```python
from build123d import *

# Parameters (mm, degrees)
BOSS_EXTRUDE1_DEPTH = 3


with BuildPart() as part:
    # Sketch1 → Boss-Extrude1 (new body)
    with BuildSketch(Plane.XY):
        Polygon((-70, -236), (70, -236), (70, -233), (56.25, -88), (56.25, 45), (-56.25, 45), (-56.25, -88), (-70, -233), align=None)
        with BuildLine():
            Line((40, -16), (-40, -16))
            ThreePointArc((-40, -16), (-45, -21), (-40, -26))
            Line((-40, -26), (40, -26))
            ThreePointArc((40, -26), (45, -21), (40, -16))
        make_face(mode=Mode.SUBTRACT)
        with BuildLine():
            Line((25, 15), (25, 25))
            Line((25, 25), (-25, 25))
            Line((-25, 25), (-25, 15))
            Line((-25, 15), (-4, 15))
            Line((-4, 15), (-4, 0))
            ThreePointArc((-4, 0), (0, -4), (4, 0))
            Line((4, 0), (4, 15))
            Line((4, 15), (25, 15))
        make_face(mode=Mode.SUBTRACT)
        with BuildLine():
            Line((40, -41), (-40, -41))
            ThreePointArc((-40, -41), (-52, -53), (-40, -65))
            Line((-40, -65), (40, -65))
            ThreePointArc((40, -65), (52, -53), (40, -41))
        make_face(mode=Mode.SUBTRACT)
        with BuildLine():
            Line((40, -80), (-40, -80))
            ThreePointArc((-40, -80), (-52, -92), (-40, -104))
            Line((-40, -104), (40, -104))
            ThreePointArc((40, -104), (52, -92), (40, -80))
        make_face(mode=Mode.SUBTRACT)
        with BuildLine():
            Line((40, -119), (-40, -119))
            ThreePointArc((-40, -119), (-52, -131), (-40, -143))
            Line((-40, -143), (40, -143))
            ThreePointArc((40, -143), (52, -131), (40, -119))
        make_face(mode=Mode.SUBTRACT)
        with BuildLine():
            Line((42.5, -158), (-42.5, -158))
            ThreePointArc((-42.5, -158), (-54.5, -170), (-42.5, -182))
            Line((-42.5, -182), (42.5, -182))
            ThreePointArc((42.5, -182), (54.5, -170), (42.5, -158))
        make_face(mode=Mode.SUBTRACT)
        with BuildLine():
            Line((45, -197), (-45, -197))
            ThreePointArc((-45, -197), (-57, -209), (-45, -221))
            Line((-45, -221), (45, -221))
            ThreePointArc((45, -221), (57, -209), (45, -197))
        make_face(mode=Mode.SUBTRACT)
    extrude(amount=BOSS_EXTRUDE1_DEPTH)


solid = part.part
```
Geometry check sheet. Reference: the model listing, model coordinates, mm. A direction names the side the tool comes from. Coordinates: 2 decimals unless noted, no trailing zeros. Loops run counter-clockwise (first coordinate to the right, second up) from the corner with the lowest first, then second, coordinate; pieces in that order, holes last. Notation, with made-up numbers: (29, 32) - (74, 32) arc R16 ccw to (74, 55) - close; hole circle Ø8 at (14.25, -0.75). An arc over 180 degrees is marked (long way). One line per item, written item: value. Start each with the question number.
(1) Depth check by flat-ended pin: P1, Ø0.9, axis at y = 22.5, z = 2, coming from the -X side. Enter the tip coordinate at first touch or a pass-through.
(2) Mould release check, pull along X, two halves, no side actions. Record for faces 1 (the cylindrical face through (52, -131, 1)), 2 (the flat face through (-1, -31, 3)), 3 (the flat face through (63.22, -161.51, 1.48)): released by +X, released by -X, zero draft, split by the parting line, or undercut.
(3) Tool access check on faces 4 (the flat face through (-63.03, -159.49, 1.48)), 5 (the cylindrical face through (-52, -92, 1)). Record the directions out of +Z, -Z, +X, -X, +Y, -Y that give a thin tool (end or side, any length) a straight path to the whole face; none if there is none.
(4) Cross-section at B-B on z = 2.3. Count the separate pieces of the cut face and the enclosed holes in it, plus the area to 3 significant figures.
(5) Cross-section at D-D on y = -33. Enter the section's corners in (x, z).
(6) Cross-section at C-C on y = -131. Enter the section's corners in (x, z).
(7) Material ranges on line 1 (Y direction, x = 47, z = 2.7); line 2 (Y direction, x = 51, z = 2.2); line 3 (X direction, y = -159, z = 2.3), recorded low to high. Write a range as [from, to].
(8) Cross-section at A-A on y = 8.5. Enter the section's corners in (x, z), plus the area to 4 significant figures.
Results below:
1. P1: stops at x = -56.25
2. face 1: undercut
2. face 2: zero draft
2. face 3: released by +X
3. face 4: +Z, -Z, -X, +Y
3. face 5: +Z, -Z
4. separate pieces: 1
4. enclosed holes: 7
4. area: 19,900 mm2
5. outline: (-56.25, 0) - (56.25, 0) - (56.25, 3) - (-56.25, 3) - close
6. outline: (-60.33, 0) - (-52, 0) - (-52, 3) - (-60.33, 3) - close; (52, 0) - (60.33, 0) - (60.33, 3) - (52, 3) - close
7. line 1: y = [-236, -220.83], [-197.17, -181.12], [-158.88, -140.75], [-121.25, -101.75], [-82.25, -62.75], [-43.25, 45]
7. line 2: y = [-236, -219.39], [-198.61, -178.47], [-161.53, -135.8], [-126.2, -96.8], [-87.2, -57.8], [-48.2, 45]
7. line 3: x = [-62.98, -47.3], [47.3, 62.98]
8. outline: (-56.25, 0) - (-4, 0) - (-4, 3) - (-56.25, 3) - close; (4, 0) - (56.25, 0) - (56.25, 3) - (4, 3) - close
8. area: 313.5 mm2
